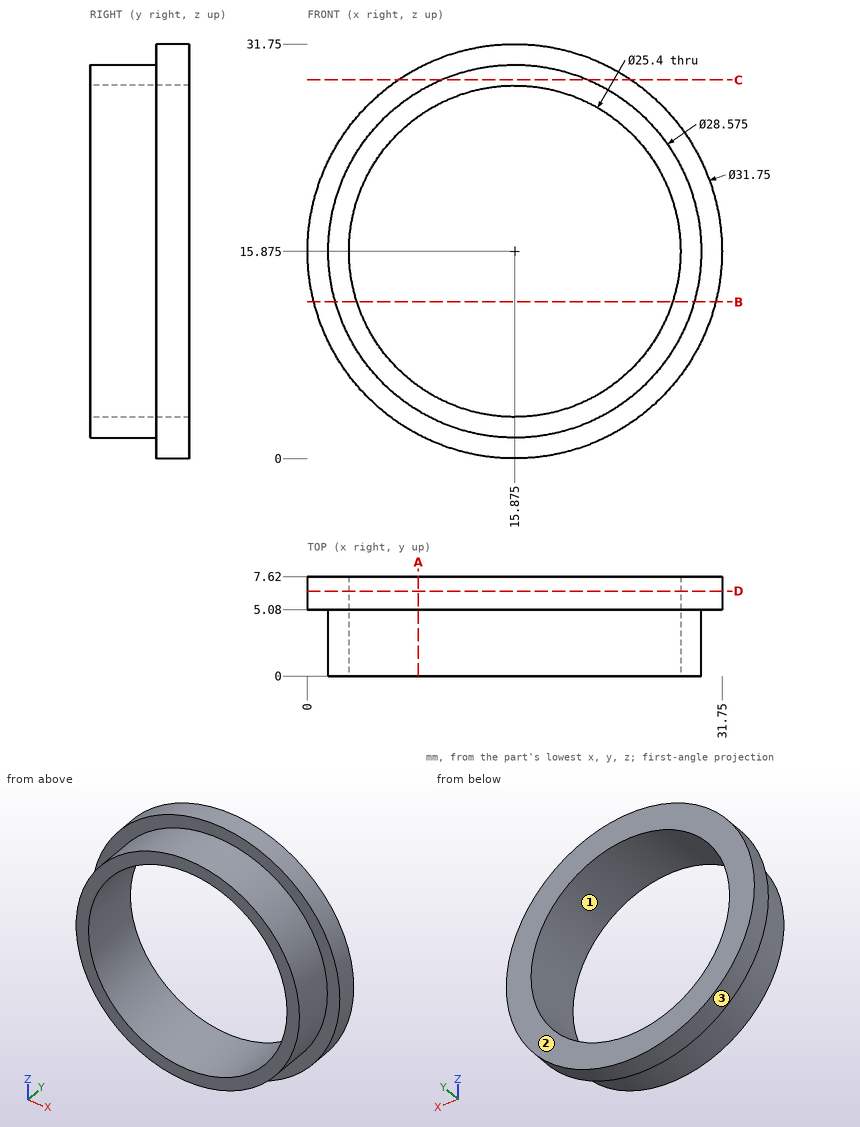
Check sheet for the drawn part. Datum: minimum x, y, z corner. Units: mm. Round coordinates to 2 decimals unless told otherwise and drop trailing zeros. Order: outer loops, then holes, each group sorted by start corner. A loop starts at its lowest first (then second) coordinate and runs counter-clockwise, first axis right, second up. Notation, with made-up numbers: (-3, -3.5) - (6, -3.5) arc R24 ccw to (6, 15.5) - close; hole circle Ø2 at (29.25, 44.5). An arc over 180 degrees is marked (long way). Use a Markdown table: item, result. Add a question column.
(1) Material ranges on line 1 along X through (y, z) = (5, 24); line 2 along Z through (x, y) = (21.5, 4.75); line 3 along Z through (x, y) = (9, 4), recorded low to high. Write a range as [from, to].
(2) Sectioned sample at A-A, the plane x = 8.5. Enter the section's corners in (y, z).
(3) Release check for a two-part mould opening along X. For the marked faces 1, 2 and 3 record: pulls with the +X half, pulls with the -X half, needs draft (parallel to the pull), parting line crosses it, or undercut.
(4) Sectioned sample at C-C, the plane z = 29. Enter the section's corners in (x, y).
(5) Sectioned sample at D-D, the plane y = 6.5. Enter the section's corners in (x, z) (3 decimals).
(6) Depth check by flat-ended pin: pin 1 (1 mm diameter, centred on y = 6.5, z = 11.5, fed in from +X). Enter the tip coordinate at first touch or a pass-through.
(7) Sectioned sample at B-B, the plane z = 12. Enter the section's corners in (x, y).
Answers below:
| question | item | result |
|---|---|---|
| 1 | line 1 | [4.12, 6.11], [25.64, 27.63] |
| 1 | line 2 | [2.74, 4.49], [27.26, 29.01] |
| 1 | line 3 | [3.35, 5.2], [26.55, 28.4] |
| 2 | outline | (0, 3.64) - (5.08, 3.64) - (5.08, 1.82) - (7.62, 1.82) - (7.62, 5.54) - (0, 5.54) - close; (0, 26.21) - (7.62, 26.21) - (7.62, 29.93) - (5.08, 29.93) - (5.08, 28.11) - (0, 28.11) - close |
| 3 | face 1 | undercut |
| 3 | face 2 | needs draft |
| 3 | face 3 | parting line crosses it |
| 4 | outline | (6.94, 5.08) - (10.23, 5.08) - (10.23, 0) - (21.52, 0) - (21.52, 5.08) - (24.81, 5.08) - (24.81, 7.62) - (6.94, 7.62) - close |
| 5 | outline | circle Ø31.75 at (15.875, 15.875); hole circle Ø25.4 at (15.875, 15.875) |
| 6 | pin 1 | x = 31.27 |
| 7 | outline | (0.48, 5.08) - (2.12, 5.08) - (2.12, 0) - (3.78, 0) - (3.78, 7.62) - (0.48, 7.62) - close; (27.97, 0) - (29.63, 0) - (29.63, 5.08) - (31.27, 5.08) - (31.27, 7.62) - (27.97, 7.62) - close |
